Autodesk Inventor part; units mm, degrees
sketch "Эскиз5" plane through (0, 0, 0) normal (0, 1, 0) x (-1, 0, 0)
  circle A0 centre (0, 0) radius 16
  dimension "d12" = 32
extrude "Выдавливание4" add sketch "Эскиз5" along normal blind 1
sketch "Эскиз7" plane through (0, 1, 0) normal (0, 1, 0) x (1, 0, 0)
  circle A0 centre (0, 0) radius 16
  circle A1 centre (0, 0) radius 16
  circle A2 centre (0, 0) radius 15
  line L0 (0.5, -14) -> (-0.5, -14)
  line L1 (-0.5, 14) -> (0.5, 14)
  line L2 (0.5, -14) -> (-0.5, 14) construction
  line L3 (-0.5, -14) -> (0.5, 14) construction
  line L4 (-0.5, -14) -> (0.5, -14)
  line L5 (0.5, -14) -> (0.5, -15.4866)
  line L6 (0.5, -15.4866) -> (-0.5, -15.4866)
  line L7 (-0.5, -15.4866) -> (-0.5, -14)
  line L8 (0.5, 14) -> (-0.5, 14)
  line L9 (-0.5, 14) -> (-0.5, 15.7701)
  line L10 (-0.5, 15.7701) -> (0.5, 15.7701)
  line L11 (0.5, 15.7701) -> (0.5, 14)
  dimension "d17" = 1
  dimension "d18" = 28
  dimension "d19" = 32
  dimension "d20" = 30
  dimension "d21" = 2.045
  dimension "d22" = 177.955
  dimension "d23" = 0
  dimension "d24" = 1.7701
  dimension "d25" = 31.2568
  dimension "d26" = 0.5
  dimension "d27" = 15.7701
extrude "Выдавливание5" add sketch "Эскиз7" along normal blind 40 contours A0 | L11 L1 L9 A2 | A2 L9 L10 L11 | L5 L6 L7 A2 | A2 L7 L0 L5
properties part number "Корпус для оборудования"
The listing builds one solid part. Answer for the finished solid, in the listing's coordinates (mm). A direction names the side the tool comes from. Coordinates: 2 decimals unless noted, no trailing zeros. Use a Markdown table: item, result. Add a question column.
1) For faces 1 (the flat face through (-0.5, 20.7, -14.5)), 2 (the flat face through (0, 0, 0)), determine the directions among +Z, -Z, +X, -X, +Y, -Y from which every point of the face is accessible in a straight line to the end or side of a thin tool.
2) Given pin 1 (1 mm diameter, centred on y = 11, z = 6.5, fed in from -X); pin 2 (5 mm diameter, centred on x = 6.5, y = 18, fed in from -Z); pin 3 (1.5 mm diameter, centred on y = 32.5, z = -2, fed in from -X), each flat-ended and moving along its own axis, determine where each tip first touches the part or whether it passes through.
3) Find the intervals of material crossed by line 1 (X direction, y = 14.5, z = 0); line 2 (Z direction, x = 0, y = 36.5); line 3 (Y direction, x = 13.5, z = 2), in increasing order.
Here are the results:
| question | item | result |
|---|---|---|
| 1 | face 1 | +Y |
| 1 | face 2 | +Z, -Z, +X, -X, -Y |
| 2 | pin 1 | stops at x = -14.83 |
| 2 | pin 2 | stops at z = -15.49 |
| 2 | pin 3 | stops at x = -15.95 |
| 3 | line 1 | x = -16 to -15, 15 to 16 |
| 3 | line 2 | z = -16 to -14, 14 to 16 |
| 3 | line 3 | y = 0 to 1 |
